Geometry check sheet. Reference: the model listing, model coordinates, mm. A direction names the side the tool comes from. Give positions to 0.01 mm unless a question says otherwise; leave off trailing zeros. Order: outer loops, then holes, each group sorted by start corner. A loop starts at its lowest first (then second) coordinate and runs counter-clockwise, first axis right, second up. Notation, with made-up numbers: M -10,-0.5 L 23,-0.5 A23 cw 23,22.5 Z; hole C 24,-22.75 d3. An arc over 180 degrees is marked long. Use CSV: the item, a comma, the result in double quotes. Start each with the question number.
from build123d import *

# Parameters (mm, degrees)
SKETCH_1_W          = 43
SKETCH_1_H          = 40.2
EXTRUDE_1_DEPTH     = 3.2
SKETCH_2_W          = 3.2
SKETCH_2_H          = 40.2
EXTRUDE_2_DEPTH     = 43.8
SKETCH_3_R          = 1.5
CUT_EXTRUDE_1_DEPTH = 43.8
CUT_EXTRUDE_2_DEPTH = 43.8
FILLET_1_R          = 2
FILLET_2_R          = 2
SKETCH_5_R          = 1.75
CUT_EXTRUDE_3_DEPTH = 43.8
FILLET_3_R          = 2


with BuildPart() as part:
    # 草图1 → 凸台-拉伸1 (new body)
    with BuildSketch(Plane(origin=(0, 0, 0), x_dir=(1, 0, 0), z_dir=(0, 1, 0))):
        Rectangle(SKETCH_1_W, SKETCH_1_H)
    extrude(amount=EXTRUDE_1_DEPTH)

    # 草图2 → 凸台-拉伸2 (add)
    with BuildSketch(Plane(origin=(0, 3.2, 0), x_dir=(1, 0, 0), z_dir=(0, 1, 0))):
        with Locations((-19.9, 0)):
            Rectangle(SKETCH_2_W, SKETCH_2_H)
    extrude(amount=EXTRUDE_2_DEPTH)

    # 草图3 → 切除-拉伸1 (cut)
    with BuildSketch(Plane.ZY.offset(21.5)):
        with Locations((-15.5, 27)):
            Circle(SKETCH_3_R)
        with Locations((-7.75, 40.423393759)):
            Circle(SKETCH_3_R)
        with Locations((7.75, 40.423393759)):
            Circle(SKETCH_3_R)
        with Locations((15.5, 27)):
            Circle(SKETCH_3_R)
        with Locations((7.75, 13.576606241)):
            Circle(SKETCH_3_R)
        with Locations((-7.75, 13.576606241)):
            Circle(SKETCH_3_R)
        with BuildLine():
            Line((-6.5, 34), (-6.5, 20))
            ThreePointArc((-6.5, 20), (0, 13.5), (6.5, 20))
            Line((6.5, 20), (6.5, 34))
            ThreePointArc((6.5, 34), (0, 40.5), (-6.5, 34))
        make_face()
    extrude(amount=-CUT_EXTRUDE_1_DEPTH, mode=Mode.SUBTRACT)

    # 草图4 → 切除-拉伸2 (cut)
    with BuildSketch(Plane.ZY.offset(21.5)):
        with BuildLine():
            Line((-20.1, 47), (-20.1, 26.9))
            ThreePointArc((-20.1, 26.9), (-14.21284635, 41.112846253), (-1.37e-07, 47))
            Line((-1.37e-07, 47), (-20.1, 47))
        make_face()
        with BuildLine():
            ThreePointArc((-1.37e-07, 47), (14.212846253, 41.11284635), (20.1, 26.9))
            Line((20.1, 26.9), (20.1, 47))
            Line((20.1, 47), (-1.37e-07, 47))
        make_face()
    extrude(amount=-CUT_EXTRUDE_2_DEPTH, mode=Mode.SUBTRACT)

    # 圆角1
    fillet_1_edges = [part.edges().sort_by_distance(p)[0] for p in [
        (-21.5, 0, 0),
    ]]
    fillet(fillet_1_edges, radius=FILLET_1_R)

    # 圆角2
    fillet_2_edges = [part.edges().sort_by_distance(p)[0] for p in [
        (-18.3, 3.2, 0),
    ]]
    fillet(fillet_2_edges, radius=FILLET_2_R)

    # 草图5 → 切除-拉伸3 (cut)
    with BuildSketch(Plane(origin=(0, 3.2, 0), x_dir=(1, 0, 0), z_dir=(0, 1, 0))):
        with Locations(Location((13.45, 14.85, 0), (0, 0, 270))):
            Circle(SKETCH_5_R)
        with Locations(Location((13.45, -15.15, 0), (0, 0, 270))):
            Circle(SKETCH_5_R)
        with Locations(Location((-10.75, -15.15, 0), (0, 0, 270))):
            Circle(SKETCH_5_R)
        with Locations(Location((-10.75, 14.85, 0), (0, 0, 270))):
            Circle(SKETCH_5_R)
    extrude(amount=-CUT_EXTRUDE_3_DEPTH, mode=Mode.SUBTRACT)

    # 圆角3
    fillet_3_edges = [part.edges().sort_by_distance(p)[0] for p in [
        (21.5, 1.6, -20.1),
        (21.5, 1.6, 20.1),
    ]]
    fillet(fillet_3_edges, radius=FILLET_3_R)


solid = part.part
(1) Sectioned sample at D-D on z = 15.15. Record the cut outline in (x, y), then the cut area to 3 significant figures.
(2) Sectioned sample at B-B on y = 23.5. Record the cut outline in (x, z), then the cut area to 3 significant figures.
(3) Sectioned sample at A-A on x = 13.45. Record the cut outline in (y, z), then the cut area to 3 significant figures.
(4) Go/stop test with flat-tipped pins: P1, Ø3, axis at x = 13.45, z = 15.15, coming from the +Y side; P2, Ø5.5, axis at x = 13.45, z = -14.85, coming from the +Y side; P3, Ø1, axis at y = 19, z = -15.5, coming from the +X side. Record where each tip stops, or that it passes through.
(5) Thickness scan on line 1 (X direction, y = 2, z = 15); line 2 (X direction, y = 1, z = -14); line 3 (X direction, y = 5, z = -18). Record the ranges inside material, lowest first.
(6) Draft check along Y on faces 4 (the face through (-18.3, 26, 9)), 5 (the face through (-19.922, 28.487, -15.695)), 6 (the face through (1, 0, 0)). Enter one of: +Y half, -Y half, draft (parallel to the pull), parting line (faces both ways), or undercut.
(7) Access from +Z, -Z, +X, -X, +Y, -Y to the whole of each face (thin tool, end or side, straight path). Record for faces 1 (the face through (21.5, 2, 0)), 2 (the face through (-19.9, 40.5, 0.1)), 3 (the face through (2, 3.2, 0)).
(8) Sectioned sample at C-C on z = 5.5. Record the cut outline in (x, y), then the cut area to 3 significant figures.
Responses:
1,outline,"M -21.5,2 A2 ccw -19.5,0 L -12.5,0 L -12.5,3.2 L -16.3,3.2 A2 cw -18.3,5.2 L -18.3,25.54 L -21.5,25.54 Z; M -21.5,28.46 L -18.3,28.46 L -18.3,40.11 L -21.5,40.11 Z; M -9,0 L 11.7,0 L 11.7,3.2 L -9,3.2 Z; M 15.2,0 L 21.5,0 L 21.5,3.2 L 15.2,3.2 Z"
1,area,"224 mm2"
2,outline,"M -21.5,-20.1 L -18.3,-20.1 L -18.3,-6.5 L -21.5,-6.5 Z; M -21.5,6.5 L -18.3,6.5 L -18.3,20.1 L -21.5,20.1 Z"
2,area,"87.0 mm2"
3,outline,"M 0,-20.1 L 3.2,-20.1 L 3.2,-16.6 L 0,-16.6 Z; M 0,-13.1 L 3.2,-13.1 L 3.2,13.4 L 0,13.4 Z; M 0,16.9 L 3.2,16.9 L 3.2,20.1 L 0,20.1 Z"
3,area,"106 mm2"
4,P1,"through"
4,P2,"y = 3.2"
4,P3,"x = -18.3"
5,line 1,"-21.5 to -12.49, -9.01 to 11.71, 15.19 to 21.5"
5,line 2,"-21.23 to -12.28, -9.22 to 11.92, 14.98 to 21.5"
5,line 3,"-21.5 to -18.29"
6,face 4,"draft"
6,face 5,"undercut"
6,face 6,"-Y half"
7,face 1,"+Z, -Z, +X, +Y, -Y"
7,face 2,"+X, -X"
7,face 3,"+Z, -Z, +X, +Y"
8,outline,"M -21.5,2 A2 ccw -19.5,0 L 21.5,0 L 21.5,3.2 L -16.3,3.2 A2 cw -18.3,5.2 L -18.3,16.54 L -21.5,16.54 Z; M -21.5,37.46 L -18.3,37.46 L -18.3,46.23 L -21.5,46.23 Z"
8,area,"208 mm2"
